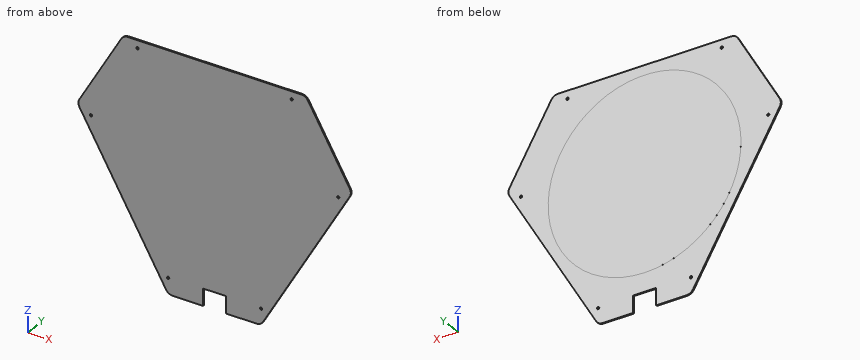
from build123d import *

# Parameters (mm, degrees)
EXTRUDE_385_DEPTH   = 1.6
FILLET_1_R          = 10
SKETCH_2_W          = 30
SKETCH_2_H          = 22
CUT_EXTRUDE_1_DEPTH = 246.888122157
SKETCH_3_R          = 125
EXTRUDE_1240_DEPTH  = 0.01
HOLE_WIZARD_3_D     = 3


with BuildPart() as part:
    # Эскиз1 → Extrude 385 (new body)
    with BuildSketch(Plane(origin=(0, 0, 0), x_dir=(1, 0, 0), z_dir=(0, 1, 0))):
        Polygon((178.156986041, -33.576951546), (60, 171.076951546), (-60, 171.076951546), (-178.156986041, -33.576951546), (-118.156986041, -137.5), (118.156986041, -137.5), align=None)
    extrude(amount=EXTRUDE_385_DEPTH)

    # Скругление1
    fillet_1_edges = [part.edges().sort_by_distance(p)[0] for p in [
        (118.156986041, 0.8, 137.5),
        (-118.156986041, 0.8, 137.5),
        (-178.156986041, 0.8, 33.576951546),
        (-60, 0.8, -171.076951546),
        (60, 0.8, -171.076951546),
        (178.156986041, 0.8, 33.576951546),
    ]]
    fillet(fillet_1_edges, radius=FILLET_1_R)

    # Эскиз2 → Вырез-Вытянуть1 (cut, through all)
    with BuildSketch(Plane(origin=(0, 1.6, 0), x_dir=(1, 0, 0), z_dir=(0, 1, 0))):
        with Locations((0, 160.076951546)):
            Rectangle(SKETCH_2_W, SKETCH_2_H)
    extrude(amount=-CUT_EXTRUDE_1_DEPTH, mode=Mode.SUBTRACT)

    # Эскиз3 → Extrude 1240 (add)
    with BuildSketch(Plane(origin=(0, 1.6, 0), x_dir=(1, 0, 0), z_dir=(0, 1, 0))):
        with Locations(Location((0, 0, 0), (0, 0, 90))):
            Circle(SKETCH_3_R)
    extrude(amount=EXTRUDE_1240_DEPTH)

    # Отверстие 3мм (through all)
    with Locations(Plane(origin=(0, 1.6, 0), x_dir=(1, 0, 0), z_dir=(0, 1, 0))):
        with Locations((-60.25, 150.255407557), (60.25, 150.255407557), (160.25, -22.9496732), (100, -127.305734356), (-100, -127.305734356), (-160.25, -22.9496732)):
            Hole(HOLE_WIZARD_3_D / 2)


solid = part.part
Here's how the part is built. I have some questions about the finished solid (model axes, mm). Coordinates: 2 decimals unless noted, no trailing zeros. Write each loop counter-clockwise with the first axis right and the second up, starting at its lowest first coordinate (ties: lowest second). Pieces come first, ordered by that corner, then holes.
Item 1: I want a section at A-A on y = 0.6. Write out the boundary of the cut face in (x, z), and give its area (3 significant figures).
Item 2: Will these pins go through, and if not, where does the flat tip stop? pin 1 (0.8 mm diameter, centred on y = 1, z = -155, fed in from -X); pin 2 (2.5 mm diameter, centred on x = -100, z = 127.31, fed in from -Y); pin 3 (2 mm diameter, centred on x = 9, z = -69, fed in from -Y); pin 4 (1.5 mm diameter, centred on x = -118, z = 89, fed in from +Y).
Item 3: If I drill on line 1 (X direction, y = 0.6, z = -151); line 2 (Y direction, x = 17.5, z = -138.5); line 3 (Z direction, x = 100, y = 0.85), over which ranges is the centre line in solid material (lowest first)?
Findings below:
1. outline: (-175.27, 28.58) - (-62.89, -166.08) arc R10 ccw to (-54.23, -171.08) - (-15, -171.08) - (-15, -149.08) - (15, -149.08) - (15, -171.08) - (54.23, -171.08) arc R10 ccw to (62.89, -166.08) - (175.27, 28.58) arc R10 ccw to (175.27, 38.58) - (121.04, 132.5) arc R10 ccw to (112.38, 137.5) - (-112.38, 137.5) arc R10 ccw to (-121.04, 132.5) - (-175.27, 38.58) arc R10 ccw to start; hole circle Ø3 at (-160.25, 22.95); hole circle Ø3 at (-100, 127.31); hole circle Ø3 at (-60.25, -150.26); hole circle Ø3 at (60.25, -150.26); hole circle Ø3 at (100, 127.31); hole circle Ø3 at (160.25, 22.95)
1. area: 78,800 mm2
2. pin 1: stops at x = -69.51
2. pin 2: passes through
2. pin 3: stops at y = 0
2. pin 4: stops at y = 1.6
3. line 1: x = -71.59 to -61.55, -58.95 to -15, 15 to 58.95, 61.55 to 71.59
3. line 2: y = 0 to 1.6
3. line 3: z = -101.79 to 125.81, 128.81 to 137.5
